Design review of the part built by this model. Coordinates are the model's own, in mm. Face numbers are marked on the shaded views. A direction names the side the tool comes from. Give positions to 0.01 mm unless a question says otherwise; leave off trailing zeros. Write each loop counter-clockwise with the first axis right and the second up, starting at its lowest first coordinate (ties: lowest second). Pieces come first, ordered by that corner, then holes. Notation, with made-up numbers: (-37, 37.5) -> (6, 37.5) arc R29 ccw to (6, 58.5) -> close; hole circle Ø11 at (41, 51.25). An arc over 180 degrees is marked (long way). Answer as a JSON object with one key per item and string values.
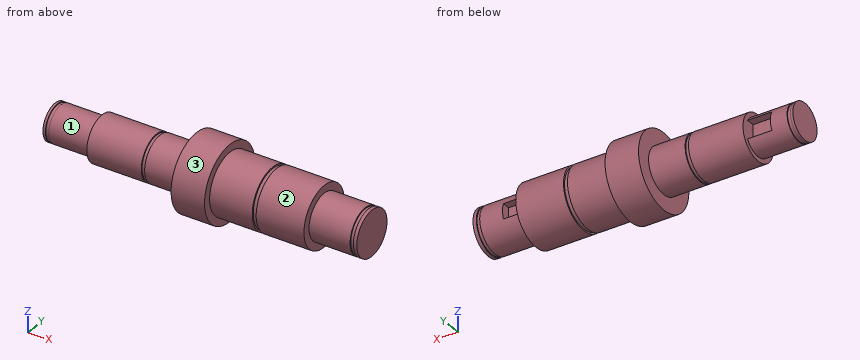
```python
from build123d import *

# Parameters (mm, degrees)
SKETCH3_W          = 6
SKETCH3_H          = 3.5
CUT_EXTRUDE1_DEPTH = 8
SKETCH4_W          = 5
SKETCH4_H          = 3
CUT_EXTRUDE3_DEPTH = 6


with BuildPart() as part:
    # Sketch1 → Revolve1 (revolve)
    with BuildSketch(Plane.XY):
        Polygon((-52.05, 0), (52.05, 0), (52.05, 7.5), (50.95, 7.5), (50.95, 7.15), (49.85, 7.15), (49.85, 7.5), (36.35, 7.5), (36.35, 10), (20.65, 10), (20.65, 9.5), (19.35, 9.5), (19.35, 10), (5.35, 10), (5.35, 12.5), (-5.65, 12.5), (-5.65, 7.5), (-17.65, 7.5), (-17.65, 7.15), (-18.75, 7.15), (-18.75, 7.5), (-36.65, 7.5), (-36.65, 6), (-50.15, 6), (-50.15, 5.75), (-51.25, 5.75), (-51.25, 6), (-52.05, 6), align=None)
    revolve(axis=Axis((-52.05, 0, 0), (1, 0, 0)))

    # Sketch3 → Cut-Extrude1 (cut)
    with BuildSketch(Plane.ZY.offset(36.65)):
        with Locations((0, 4.25)):
            Rectangle(SKETCH3_W, SKETCH3_H)
    extrude(amount=CUT_EXTRUDE1_DEPTH, mode=Mode.SUBTRACT)

    # Sketch4 → Cut-Extrude3 (cut)
    with BuildSketch(Plane(origin=(36.35, 0, 0), x_dir=(0, 0, -1), z_dir=(1, 0, 0))):
        with Locations((0, 6)):
            Rectangle(SKETCH4_W, SKETCH4_H)
    extrude(amount=CUT_EXTRUDE3_DEPTH, mode=Mode.SUBTRACT)


solid = part.part
```
(1) For the marked faces 1, 2 and 3, list the 3-axis set-ups (+Z, -Z, +X, -X, +Y, -Y) from which the entire face can be reached by the end or side of a thin tool; tool diameter is ignored.
Here are the results:
{"face 1": "-X", "face 2": "+X", "face 3": "+X, -X"}
(2) We need section B-B, the plane z = -11. State the section outline as (x, y) points.
Here are the results:
{"outline": "(-5.65, -5.94) -> (5.35, -5.94) -> (5.35, 5.94) -> (-5.65, 5.94) -> close"}
(3) We need section C-C, the plane x = -1. State the section outline as (y, z) points, then the cut area to 3 significant figures.
Here are the results:
{"outline": "circle Ø25 at (0, 0)", "area": "491 mm²"}
(4) We need section D-D, the plane x = 39. State the section outline as (y, z) points.
Here are the results:
{"outline": "(4.5, -2.5) -> (4.5, 2.5) -> (7.07, 2.5) arc R7.5 ccw (long way) to (7.07, -2.5) -> close"}
(5) Clearance check with flat-ended pins moving along their axes: pin 1 (2 mm diameter, centred on x = -41, y = 4.5, fed in from -Z); pin 2 (4 mm diameter, centred on x = 32, z = 3.5, fed in from -Y); pin 3 (1 mm diameter, centred on x = -40.5, y = -3.5, fed in from +Z). State where each tip first meets the part, or that it passes through.
Here are the results:
{"pin 1": "stops at z = -4.87", "pin 2": "stops at y = -9.89", "pin 3": "stops at z = 5.2"}
(6) For line 1 along X through (y, z) = (-3.75, 6.25); line 2 along X through (y, z) = (3, -2.25); line 3 along X through (y, z) = (-3.5, -9), list the stretches that pass through material, from the lowest coordinate up.
Here are the results:
{"line 1": "x = -36.65 to -18.75, -17.65 to 49.85, 50.95 to 52.05", "line 2": "x = -52.05 to -44.65, -36.65 to 52.05", "line 3": "x = -5.65 to 19.35, 20.65 to 36.35"}
(7) We need section A-A, the plane x = -31.5. State the section outline as (y, z) points.
Here are the results:
{"outline": "circle Ø15 at (0, 0)"}
